Here's the drawing with two shaded views (mm, measured from the low corner). I have some questions. Coordinates: 2 decimals unless noted, no trailing zeros. Order: outer loops, then holes, each group sorted by start corner. A loop starts at its lowest first (then second) coordinate and runs counter-clockwise, first axis right, second up. Notation, with made-up numbers: (-14, -26.75) -> (10, -26.75) arc R32 cw to (10, 2.25) -> close; hole circle Ø2 at (89, -8.5). An arc over 180 degrees is marked (long way). Answer as a JSON object with one key per item and string values. Group by question number.
(1) I want a section at B-B, the plane x = 40. List the corners of the cut face in (y, z) for me, plus the area to 3 significant figures.
(2) I need wall thicknesses on line 1 (Y direction, x = 7.5, z = 1.1); line 2 (X direction, y = 7.5, z = 1.65); line 3 (Z direction, x = 33, y = 33). Which ranges of each line are inside material? Lowest first, please.
(3) I want a section at C-C, the plane y = 25. List the corners of the cut face in (x, z) for me, plus the area to 3 significant figures.
(4) If we mould it in two halves opening along Z, with no side actions, what happens to the marked faces 1, 2 and 3? For each: pulls with the +Z half, pulls with the -Z half, needs draft (parallel to the pull), parting line crosses it, or undercut.
(5) For pin 1 (3 mm diameter, centred on x = 73, z = 4.5, fed in from -Y); pin 2 (6 mm diameter, centred on x = 72.5, y = 7.5, fed in from +Z); pin 3 (5 mm diameter, centred on y = 5.5, z = 14.5, fed in from +X); pin 4 (4 mm diameter, centred on x = 7.5, y = 7.5, fed in from -Z), each with a flat end and sliding along its axis, tell me the tip position at first contact or that it passes through.
(6) I want a section at A-A, the plane x = 7.5. List the corners of the cut face in (y, z) for me.
(7) I want a section at D-D, the plane z = 46. List the corners of the cut face in (x, y) for me (1 decimal).
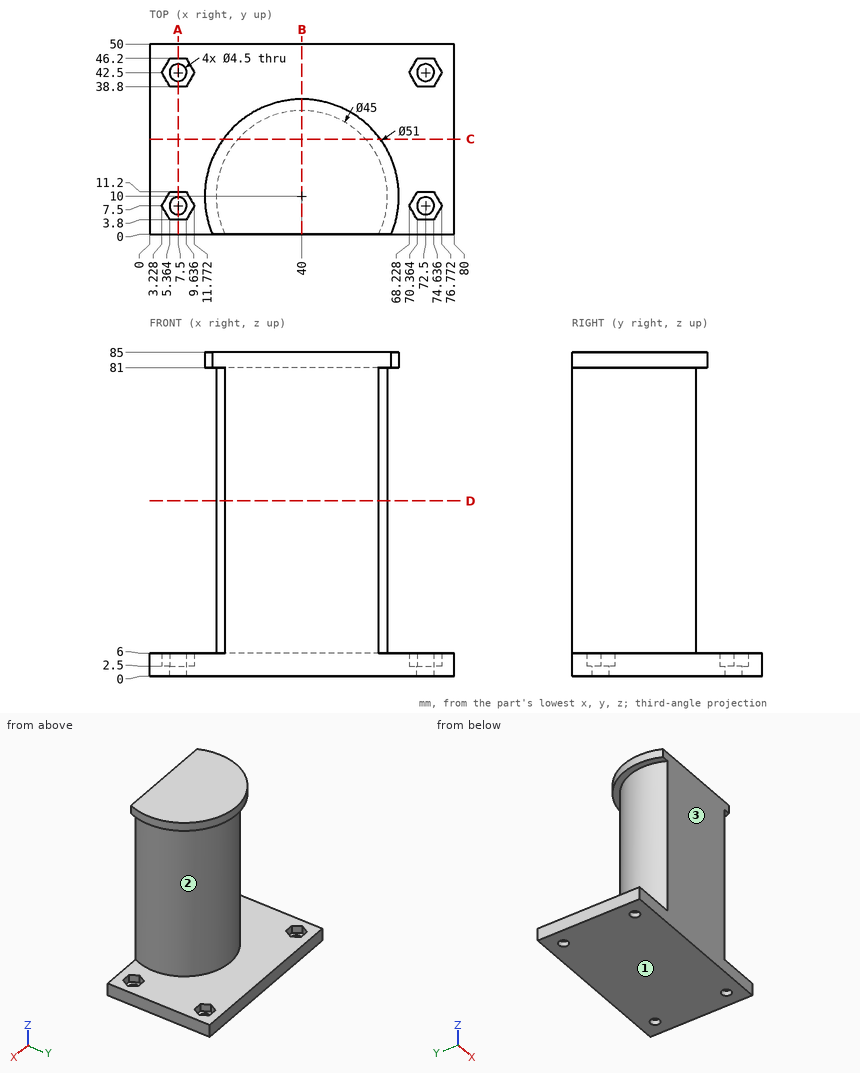
Computed values:
{
 "1": {"outline": "(0, 0) -> (50, 0) -> (50, 6) -> (32.5, 6) -> (32.5, 81) -> (35.5, 81) -> (35.5, 85) -> (0, 85) -> close", "area": "2,880 mm2"},
 "2": {"line 1": "y = 0 to 5.25, 9.75 to 40.25, 44.75 to 50", "line 2": "x = 0 to 5.25, 9.75 to 70.25, 74.75 to 80", "line 3": "z = 0 to 6, 81 to 85"},
 "3": {"outline": "(0, 0) -> (80, 0) -> (80, 6) -> (56.77, 6) -> (56.77, 81) -> (60.62, 81) -> (60.62, 85) -> (19.38, 85) -> (19.38, 81) -> (23.23, 81) -> (23.23, 6) -> (0, 6) -> close", "area": "3,160 mm2"},
 "4": {"face 1": "pulls with the -Z half", "face 2": "undercut", "face 3": "needs draft"},
 "5": {"pin 1": "stops at y = 0", "pin 2": "stops at z = 2.5", "pin 3": "stops at x = 62.41", "pin 4": "passes through"},
 "6": {"outline": "(0, 0) -> (5.25, 0) -> (5.25, 2.5) -> (3.8, 2.5) -> (3.8, 6) -> (0, 6) -> close; (9.75, 0) -> (40.25, 0) -> (40.25, 2.5) -> (38.8, 2.5) -> (38.8, 6) -> (11.2, 6) -> (11.2, 2.5) -> (9.75, 2.5) -> close; (44.75, 0) -> (50, 0) -> (50, 6) -> (46.2, 6) -> (46.2, 2.5) -> (44.75, 2.5) -> close"},
 "7": {"outline": "(19.8, 0) -> (60.2, 0) arc R22.5 ccw (long way) to start"}
}
